Job drawing, mm, ordinate dimensions from the low corner. One solid piece. A direction names the side the tool comes from. Give positions to 0.01 mm unless a question says otherwise; leave off trailing zeros. Order: outer loops, then holes, each group sorted by start corner. A loop starts at its lowest first (then second) coordinate and runs counter-clockwise, first axis right, second up. Notation, with made-up numbers: (29.25, 26.5) - (72.25, 26.5) arc R9 cw to (72.25, 34.5) - close; hole circle Ø9 at (73.5, -28.5). An arc over 180 degrees is marked (long way). Use a Markdown table: item, result. Add a question column.
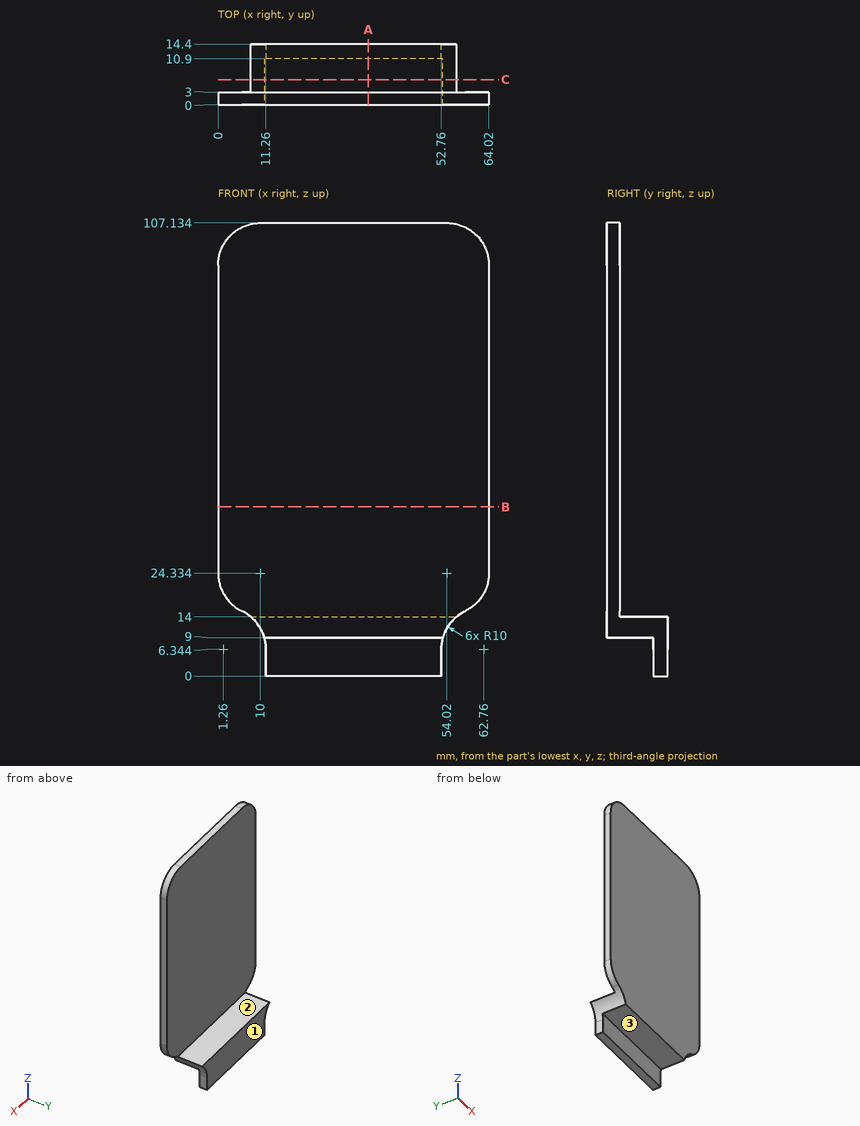
1. Cut at B-B (z = 40). Write the cut outline in (x, y), plus the area to 3 significant figures.
2. Pin check, flat tips, straight feed: P1, Ø6, axis at x = 17, z = 67, coming from the -Y side; P2, Ø4, axis at x = 50.5, y = 7, coming from the -Z side; P3, Ø4, axis at y = 12.5, z = 3.5, coming from the -X side; P4, Ø4, axis at y = 13, z = 4.5, coming from the +X side. Stop position of each tip, or through.
3. Cut at C-C (y = 6). Write the cut outline in (x, z) (1 decimal).
4. Cut at A-A (x = 35.5). Write the cut outline in (y, z).
5. Drill centre lines: probe 1 along Z at (x, y) = (50.5, 10); probe 2 along Z at (x, y) = (36.5, 0.5); probe 3 along Y at (x, z) = (15, 85.5). Where is each one in solid material? Low to high. Write a range as [from, to].
6. Tool access for the marked faces 1, 2 and 3: list every direction of +Z, -Z, +X, -X, +Y, -Y with a clear straight run to the whole face (end or side of a thin tool).
Responses:
| question | item | result |
|---|---|---|
| 1 | outline | (0, 0) - (64.02, 0) - (64.02, 3) - (0, 3) - close |
| 1 | area | 192 mm² |
| 2 | P1 | stops at y = 0 |
| 2 | P2 | stops at z = 9 |
| 2 | P3 | stops at x = 11.26 |
| 2 | P4 | stops at x = 52.76 |
| 3 | outline | (7.7, 14) arc R10 cw to (10.9, 9) - (53.1, 9) arc R10 cw to (56.3, 14) - close |
| 4 | outline | (0, 9) - (10.9, 9) - (10.9, 0) - (14.4, 0) - (14.4, 14) - (3, 14) - (3, 107.13) - (0, 107.13) - close |
| 5 | probe 1 | z = [9, 14] |
| 5 | probe 2 | z = [9, 107.13] |
| 5 | probe 3 | y = [0, 3] |
| 6 | face 1 | +Z, -Z, +X, -X, +Y |
| 6 | face 2 | +Z, +X, -X, +Y |
| 6 | face 3 | -Z, +X, -X, -Y |
